Check sheet for the modelled part. Datum: model origin and axes. Units: mm. A direction names the side the tool comes from. Give positions to 0.01 mm unless a question says otherwise; leave off trailing zeros. Loops run counter-clockwise (first coordinate to the right, second up) from the corner with the lowest first, then second, coordinate; pieces in that order, holes last. Notation, with made-up numbers: (71.25, 85.5) -> (120.25, 85.5) arc R24 ccw to (120.25, 122.5) -> close; hole circle Ø6 at (-21, 85). An arc over 180 degrees is marked (long way). Write each question's results on one line, items separated by ' | '. Start each with the question number.
1. Material ranges on L1, parallel to X at y = 2.5, z = -4.5; L2, parallel to Z at x = -3, y = 2.25; L3, parallel to Y at x = -2.25, z = 1.25, recorded low to high. Write a range as from..to.
2. Mould release check, pull along X, two halves, no side actions. Record for faces 1 (the face through (2.07, 2.41, 3.8)), 2 (the face through (0, 5, 6.5)), 3 (the face through (2.07, 5.95, -2.68)), 4 (the face through (5, 5, 0)): +X half, -X half, draft (parallel to the pull), parting line (faces both ways), or undercut.
3. Gauge pin test, flat end, axial feed: pin 1 Ø1.8 at (y, z) = (4, -2.5) entering from -X. Record the tip position at first contact, or that the pin passes through.
4. Cross-section at A-A on y = 3. Record the boundary of the cut face in (x, z), and give its area (3 significant figures).
5. Cross-section at B-B on x = -2.25. Record the boundary of the cut face in (y, z).
6. Cross-section at D-D on z = -0.5. Record the boundary of the cut face in (x, y).
7. Tool access check on faces 5 (the face through (-2, 2, 4.25)), 6 (the face through (2.5, 3, -2)), 7 (the face through (0, 10, 0)). Record the directions out of +Z, -Z, +X, -X, +Y, -Y that give a thin tool (end or side, any length) a straight path to the whole face; none if there is none.
from build123d import *

# Parameters (mm, degrees)
SKETCH1_W           = 10
SKETCH1_H           = 13
BOSS_EXTRUDE1_DEPTH = 10
SKETCH2_W           = 8.5
SKETCH2_H           = 5
CUT_EXTRUDE1_DEPTH  = 7.5
SKETCH3_W           = 3
SKETCH3_H           = 5
CUT_EXTRUDE3_DEPTH  = 10.75
FILLET3_R           = 3
FILLET5_R           = 1.5


with BuildPart() as part:
    # Sketch1 → Boss-Extrude1 (new body)
    with BuildSketch(Plane(origin=(0, 0, 0), x_dir=(1, 0, 0), z_dir=(0, 1, 0))):
        Rectangle(SKETCH1_W, SKETCH1_H)
    extrude(amount=BOSS_EXTRUDE1_DEPTH)

    # Sketch2 → Cut-Extrude1 (cut)
    with BuildSketch(Plane.ZY.offset(5)):
        with Locations((0, 3.9)):
            Rectangle(SKETCH2_W, SKETCH2_H)
    extrude(amount=-CUT_EXTRUDE1_DEPTH, mode=Mode.SUBTRACT)

    # Sketch3 → Cut-Extrude3 (cut)
    with BuildSketch(Plane(origin=(0, 0, -6.5), x_dir=(-1, 0, 0), z_dir=(0, 0, -1))):
        with Locations((-1, 3.9)):
            Rectangle(SKETCH3_W, SKETCH3_H)
    extrude(amount=-CUT_EXTRUDE3_DEPTH, mode=Mode.SUBTRACT)

    # Fillet3
    fillet3_edges = [part.edges().sort_by_distance(p)[0] for p in [
        (-1.25, 6.4, 4.25),
        (-2.75, 6.4, -4.25),
    ]]
    fillet(fillet3_edges, radius=FILLET3_R)

    # Fillet5
    fillet5_edges = [part.edges().sort_by_distance(p)[0] for p in [
        (2.5, 2.4, 4.25),
        (2.5, 5.521320344, 3.371320344),
        (2.5, 6.4, -2.625),
        (-0.5, 6.4, -3.875),
    ]]
    fillet(fillet5_edges, radius=FILLET5_R - 0.0001)  # a hair under: the kernel refuses the full size


solid = part.part
Geometry says:
1) L1: -5..-0.5, 2.5..5 | L2: -6.5..-4.25, 4.25..6.5 | L3: 0..1.4, 6.4..10
2) face 1: -X half | face 2: draft | face 3: undercut | face 4: +X half
3) pin 1: x = 2.5
4) outline: (-5, -6.5) -> (-0.5, -6.5) -> (-0.5, -4.25) -> (-5, -4.25) -> close; (-5, 4.25) -> (1, 4.25) arc R1.5 cw to (2.5, 2.75) -> (2.5, -6.5) -> (5, -6.5) -> (5, 6.5) -> (-5, 6.5) -> close | area: 60.0 mm^2
5) outline: (0, -6.5) -> (10, -6.5) -> (10, 6.5) -> (0, 6.5) -> close; hole (1.4, -4.25) -> (3.4, -4.25) arc R3 ccw to (6.4, -1.25) -> (6.4, 1.25) arc R3 ccw to (3.4, 4.25) -> (1.4, 4.25) -> close
6) outline: (-5, 0) -> (5, 0) -> (5, 10) -> (-5, 10) -> (-5, 6.4) -> (1, 6.4) arc R1.5 cw to (2.5, 4.9) -> (2.5, 1.4) -> (-5, 1.4) -> close
7) face 5: -X | face 6: -Z | face 7: +Z, -Z, +X, -X, +Y
